Can you work these out from the model? Positions are in its coordinate system, mm. Face numbers are marked on the shaded views. A direction names the side the tool comes from. Round coordinates to 2 decimals unless told otherwise and drop trailing zeros. Loops run counter-clockwise (first coordinate to the right, second up) from the corner with the lowest first, then second, coordinate; pieces in that order, holes last. Notation, with made-up numbers: (42, 52) -> (101, 52) arc R19 cw to (101, 75) -> close; hole circle Ø11 at (38.25, -29). An arc over 180 degrees is marked (long way). Write item = value, one per line.
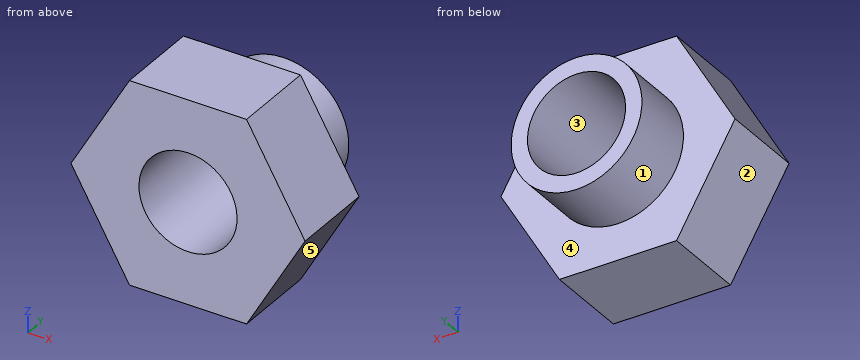
from build123d import *

# Parameters (mm, degrees)
SKETCH1_R           = 50
BOSS_EXTRUDE1_DEPTH = 65
SKETCH1_3_R         = 50
BOSS_EXTRUDE2_DEPTH = 115
SKETCH1_4_R         = 37.5
CUT_EXTRUDE1_DEPTH  = 115


with BuildPart() as part:
    # Sketch1 → Boss-Extrude1 (new body)
    with BuildSketch(Plane(origin=(0, 0, 0), x_dir=(1, 0, 0), z_dir=(0, 1, 0))):
        Polygon((-44.744645862, -77.5), (44.744645862, -77.5), (89.489291724, 0), (44.744645862, 77.5), (-44.744645862, 77.5), (-89.489291724, 0), align=None)
        with Locations(Location((0, 0, 0), (0, 0, 270))):
            Circle(SKETCH1_R, mode=Mode.SUBTRACT)
    extrude(amount=BOSS_EXTRUDE1_DEPTH)

    # Sketch1_3 → Boss-Extrude2 (add)
    with BuildSketch(Plane(origin=(0, 0, 0), x_dir=(1, 0, 0), z_dir=(0, 1, 0))):
        with Locations(Location((0, 0, 0), (0, 0, 270))):
            Circle(SKETCH1_3_R)
    extrude(amount=BOSS_EXTRUDE2_DEPTH)

    # Sketch1_4 → Cut-Extrude1 (cut)
    with BuildSketch(Plane(origin=(0, 0, 0), x_dir=(1, 0, 0), z_dir=(0, 1, 0))):
        with Locations(Location((0, 0, 0), (0, 0, 270))):
            Circle(SKETCH1_4_R)
    extrude(amount=CUT_EXTRUDE1_DEPTH, mode=Mode.SUBTRACT)


solid = part.part
1. I need wall thicknesses on line 1 (X direction, y = 54, z = 0); line 2 (X direction, y = 65.5, z = 0); line 3 (Y direction, x = -32, z = 60). Which ranges of each line are inside material? Lowest first, please. Write a range as [from, to].
Entries:
line_1 = [-89.49, -37.5], [37.5, 89.49]
line_2 = [-50, -37.5], [37.5, 50]
line_3 = [0, 65]
2. Suppose I cut it at C-C, the plane z = -4.5. List the corners of the cut face in (x, y) for me, and give its area (3 significant figures).
Entries:
outline = (-86.89, 0) -> (-37.23, 0) -> (-37.23, 115) -> (-49.8, 115) -> (-49.8, 65) -> (-86.89, 65) -> close; (37.23, 0) -> (86.89, 0) -> (86.89, 65) -> (49.8, 65) -> (49.8, 115) -> (37.23, 115) -> close
area = 7,710 mm²
3. Suppose I cut it at D-D, the plane z = -45. List the corners of the cut face in (x, y) for me, and give its area (3 significant figures).
Entries:
outline = (-63.51, 0) -> (63.51, 0) -> (63.51, 65) -> (21.79, 65) -> (21.79, 115) -> (-21.79, 115) -> (-21.79, 65) -> (-63.51, 65) -> close
area = 10,400 mm²
4. We'd pull the mould along X, two halves only. Please class the marked faces 3, 4 and 5: released by +X, released by -X, zero draft, split by the parting line, or undercut.
Entries:
face_3 = undercut
face_4 = zero draft
face_5 = released by +X
5. For the marked faces 1 and 2, which set-ups out of +Z, -Z, +X, -X, +Y, -Y let a thin tool reach every point of the face, with its end or its side?
Entries:
face_1 = +Y
face_2 = -Z, -X, +Y, -Y
6. Suppose I cut it at A-A, the plane x = 0. List the corners of the cut face in (y, z) for me.
Entries:
outline = (0, -77.5) -> (65, -77.5) -> (65, -50) -> (115, -50) -> (115, -37.5) -> (0, -37.5) -> close; (0, 37.5) -> (115, 37.5) -> (115, 50) -> (65, 50) -> (65, 77.5) -> (0, 77.5) -> close
7. I'm going to push flat-ended pins straight in: pin 1 (12 mm diameter, centred on x = 15.5, y = 76, fed in from +Z); pin 2 (1.5 mm diameter, centred on x = -46, y = 31, fed in from -Z); pin 3 (1.5 mm diameter, centred on y = 73, z = -47, fed in from -X). Where does each tip first touch, or does it pass through?
Entries:
pin_1 = 49.09
pin_2 = -76.62
pin_3 = -19
8. Suppose I cut it at B-B, the plane y = 28. List the corners of the cut face in (x, z) for me.
Entries:
outline = (-89.49, 0) -> (-44.74, -77.5) -> (44.74, -77.5) -> (89.49, 0) -> (44.74, 77.5) -> (-44.74, 77.5) -> close; hole circle Ø75 at (0, 0)
